CAD build for the part. Positions are in the model's coordinates, mm. A direction names the side the tool comes from. Give positions to 0.01 mm unless a question says otherwise; leave off trailing zeros. Order: outer loops, then holes, each group sorted by start corner. A loop starts at its lowest first (then second) coordinate and runs counter-clockwise, first axis right, second up. Notation, with made-up numbers: M 5,-27.75 L 21,-27.75 A20 cw 21,-12.75 Z; hole C 35.25,65 d6. An arc over 180 degrees is marked long. Put each result on its own line as item: value. Start each with the question number.
1) Pin check, flat tips, straight feed: pin 1 (1.6 mm diameter, centred on x = 5, z = 4.5, fed in from -Y); pin 2 (0.9 mm diameter, centred on x = -0.5, y = 3, fed in from +Z); pin 3 (3 mm diameter, centred on x = 6.5, z = 0.5, fed in from -Y). Stop position of each tip, or through.
2) Tool access for faces 5 (the face through (4.075, 2, 5)), 6 (the face through (3.6, 4.8, 4.8)), 7 (the face through (3.075, 2, 5)), 8 (the face through (6.55, 2, -1)): list every direction of +Z, -Z, +X, -X, +Y, -Y with a clear straight run to the whole face (end or side of a thin tool).
3) Two-plate mould, pull along Y, no slides. Class faces 1 (the face through (2, 2.3, 5)), 2 (the face through (7, 2, -2.95)), 3 (the face through (4, 4, 2)), 4 (the face through (3.358, 1.824, -1.574)): released by +Y, released by -Y, zero draft, split by the parting line, or undercut.
4) Cut at D-D (z = 4). Write the cut outline in (x, y) (3 decimals), and give its area (3 significant figures).
5) Cut at B-B (y = 2.8). Write the cut outline in (x, z) (3 decimals), and give its area (3 significant figures).
6) Drill centre lines: line 1 (X direction, y = 2.8, z = 1.45) (3 decimals); line 2 (X direction, y = 4.75, z = -0.5); line 3 (Z direction, x = 1, y = 4.75). Where is each one in solid material? Low to high. Write a range as [from, to].
7) Cut at C-C (x = 6.75). Write the cut outline in (y, z).
8) Cut at A-A (z = 0.25). Write the cut outline in (x, y) (3 decimals).
Autodesk Fusion 360 part; units mm, degrees
sketch "Sketch1" plane through (0, 0, 0) normal (0, 1, 0) x (1, 0, 0)
  line L0 (0, 0) -> (7.15, 0)
  line L1 (7.15, 0) -> (7.15, -3.3)
  line L2 (7.15, -3.3) -> (0, -3.3)
  line L3 (0, -3.3) -> (0, 0)
  line L4 (0, 0) -> (0.6, 0)
  line L5 (0.6, 0) -> (0.6, 2.95)
  line L6 (0.6, 2.95) -> (0, 2.95)
  line L7 (0, 2.95) -> (0, 0)
  line L8 (7.15, 0) -> (6.55, 0)
  line L9 (6.55, 0) -> (6.55, 2.95)
  line L10 (6.55, 2.95) -> (7.15, 2.95)
  line L11 (7.15, 2.95) -> (7.15, 0)
  dimension "d1" = 7.15
  dimension "d2" = 3.3
  dimension "d3" = 0.6
  dimension "d4" = 2.95
  dimension "d5" = 0.6
  dimension "d6" = 2.95
extrude "Extrude1" add sketch "Sketch1" along normal blind 5.6
sketch "Sketch2" plane through (7.15, 0, 0) normal (1, 0, 0) x (0, 1, 0)
  line L0 (0, 3.3) -> (0, -2.95)
  line L1 (0, -2.95) -> (5.6, -2.95)
  line L2 (5.6, -2.95) -> (5.6, 3.3)
  line L3 (5.6, 3.3) -> (0, 3.3)
  line L4 (1.675, -2.95) -> (3.925, -2.95)
  line L5 (3.925, -2.95) -> (3.925, 2.05)
  line L6 (3.925, 2.05) -> (1.675, 2.05)
  line L7 (1.675, 2.05) -> (1.675, -2.95)
  point P0 (2.8, 0)
  dimension "d12" = 2.25
  dimension "d13" = 5
extrude "Extrude2" add sketch "Sketch2" along normal blind 0.8 contours L1 L4 L5 L6 L7
sketch "Sketch3" plane through (0, 0, 0) normal (-1, 0, 0) x (0, -1, 0)
  line L0 (0, -2.95) -> (0, 3.3)
  line L1 (0, 3.3) -> (-5.6, 3.3)
  line L2 (-5.6, 3.3) -> (-5.6, -2.95)
  line L3 (-5.6, -2.95) -> (0, -2.95)
  line L4 (-1.675, -2.5004) -> (-1.675, -2.95)
  line L5 (-1.675, -2.95) -> (-3.925, -2.95)
  line L6 (-3.925, -2.95) -> (-3.925, -2.5004)
  line L7 (-1.675, -2.95) -> (-3.925, -2.95)
  line L8 (-3.925, -2.95) -> (-3.925, 2.05)
  line L9 (-3.925, 2.05) -> (-1.675, 2.05)
  line L10 (-1.675, 2.05) -> (-1.675, -2.95)
  point P0 (-2.8, -0.0004)
  dimension "d19" = 2.25
  dimension "d20" = 5
extrude "Extrude3" add sketch "Sketch3" along normal blind 0.8 contours L3 L4 L5 L6 L7 L8 L9 L10
sketch "Sketch4" plane through (0, 0, 0) normal (0, -1, 0) x (1, 0, 0)
  line L0 (0.6, -2.95) -> (0.6, 0)
  line L1 (0.6, 0) -> (6.55, 0)
  line L2 (6.55, 0) -> (6.55, -2.95)
  line L3 (6.55, -2.95) -> (7.15, -2.95)
  line L4 (7.15, -2.95) -> (7.15, 3.3)
  line L5 (7.15, 3.3) -> (0, 3.3)
  line L6 (0, 3.3) -> (0, -2.95)
  line L7 (0, -2.95) -> (0.6, -2.95)
  line L8 (0, 0) -> (0.6, 0)
  line L9 (0.6, 0) -> (0.6, -2.95)
  line L10 (0.6, -2.95) -> (0, -2.95)
  line L11 (0, -2.95) -> (0, 0)
  line L12 (6.55, 0) -> (7.15, 0)
  line L13 (7.15, 0) -> (7.15, -2.95)
  line L14 (7.15, -2.95) -> (6.55, -2.95)
  line L15 (6.55, -2.95) -> (6.55, 0)
extrude "Extrude4" add sketch "Sketch4" along normal blind 2 contours L0 L6 L7 L8 L9 L10 L11 | L2 L3 L4 L12 L13 L14 L15
sketch "Sketch5" plane through (0, 0, 0) normal (-1, 0, 0) x (0, -1, 0)
  line L0 (-3.925, -2.95) -> (-3.925, 2.05)
  line L1 (-3.925, 2.05) -> (-1.675, 2.05)
  line L2 (-1.675, 2.05) -> (-1.675, -2.95)
  line L3 (0, 0) -> (0, 3.3)
  line L4 (0, 3.3) -> (-5.6, 3.3)
  line L5 (-5.6, 3.3) -> (-5.6, -2.95)
  line L6 (-5.6, -2.95) -> (-3.925, -2.95)
sketch "Sketch6" plane through (0, 0, -2.95) normal (0, 0, -1) x (1, 0, 0)
  line L0 (0, 2) -> (0, -1.675)
  line L1 (0, -1.675) -> (-0.8, -1.675)
  line L2 (-0.8, -1.675) -> (-0.8, -3.925)
  line L3 (-0.8, -3.925) -> (0, -3.925)
  line L4 (0, -3.925) -> (0, -5.6)
  line L5 (0, -5.6) -> (0.6, -5.6)
  line L6 (0.6, -5.6) -> (0.6, 2)
  line L7 (0.6, 2) -> (0, 2)
  line L8 (0.6, 2) -> (0, 2)
  line L9 (0, 2) -> (0, 1.4)
  line L10 (0, 1.4) -> (0.6, 1.4)
  line L11 (0.6, 1.4) -> (0.6, 2)
sketch "Sketch7" plane through (0, 0, -2.95) normal (0, 0, -1) x (1, 0, 0)
  line L0 (6.55, 2) -> (6.55, -5.6)
  line L1 (6.55, -5.6) -> (7.15, -5.6)
  line L2 (7.15, -5.6) -> (7.15, -3.925)
  line L3 (7.15, -3.925) -> (7.95, -3.925)
  line L4 (7.95, -3.925) -> (7.95, -1.675)
  line L5 (7.95, -1.675) -> (7.15, -1.675)
  line L6 (7.15, -1.675) -> (7.15, 2)
  line L7 (7.15, 2) -> (6.55, 2)
  line L8 (7.15, 2) -> (6.55, 2)
  line L9 (6.55, 2) -> (6.55, 1.4)
  line L10 (6.55, 1.4) -> (7.15, 1.4)
  line L11 (7.15, 1.4) -> (7.15, 2)
  dimension "d25" = 0.6
extrude "Extrude5" add sketch "Sketch7" sketch "Sketch6" along normal blind 0.5 contours L0 L6 L7 L8 L9 L10 L11 of sketch 2 contours L0 L6 L7 L8 L9 L10 L11
sketch "Sketch8" plane through (0, 0, 0) normal (-1, 0, 0) x (0, -1, 0)
  line L0 (0.2, 0) -> (1.25, -2.95)
  line L1 (1.25, -2.95) -> (1.3, -3.6)
  line L2 (1.3, -3.6) -> (2.5, -3.6)
  line L3 (2.5, -3.6) -> (2.5, 0.457)
  line L4 (2.5, 0.457) -> (0.2, 0)
sketch "Sketch9" plane through (0, -1.35, -1.5715) normal (-1, 0, 0) x (0, -1, 0)
extrude "Extrude6" cut sketch "Sketch8" against normal blind 11
sketch "Sketch10" plane through (0, 0, 0) normal (0, 0, -1) x (1, 0, 0)
  line L0 (6.55, 0) -> (0.6, 0)
  line L1 (0.6, 0) -> (0.6, -5.6)
  line L2 (0.6, -5.6) -> (6.55, -5.6)
  line L3 (6.55, -5.6) -> (6.55, 0)
  line L4 (3.575, -5.6) -> (3.575, 0)
  circle A0 centre (3.575, -2.8) radius 1
  circle A1 centre (3.575, -2.8) radius 2
  dimension "d30" = 2
  dimension "d31" = 4
extrude "Extrude7" cut sketch "Sketch10" against normal blind 2 contours L4 A0 A1 | L4 A0 A1
extrude "Extrude8" add 1 faces at (3.8935, 2.8983, 0) along direction (0, 0, -1) blind 5.5
sketch "Sketch11" plane through (0, 0, 0) normal (0, 1, 0) x (1, 0, 0)
fillet "Fillet1" radius 0.25 1 edges at (2.6427, 3.1616, -5.5)
sketch "Sketch12" plane through (0, 0, 3.3) normal (0, 0, 1) x (-1, 0, 0)
  line L0 (0, 0) -> (-7.15, 0)
  line L1 (-7.15, 0) -> (-7.15, -5.6)
  line L2 (-7.15, -5.6) -> (0, -5.6)
  line L3 (0, -5.6) -> (0, 0)
  line L4 (-3.575, -5.6) -> (-3.575, 0)
  line L5 (0, -2.8) -> (-7.15, -2.8)
  line L6 (-1.575, -4.8) -> (-5.575, -4.8)
  line L7 (-5.575, -4.8) -> (-5.575, -0.8)
  line L8 (-5.575, -0.8) -> (-1.575, -0.8)
  line L9 (-1.575, -0.8) -> (-1.575, -4.8)
  line L10 (-1.575, -4.8) -> (-5.575, -0.8) construction
  line L11 (-5.575, -4.8) -> (-1.575, -0.8) construction
  line L12 (-3.075, -4.8) -> (-4.075, -4.8)
  line L13 (-4.075, -4.8) -> (-4.075, -0.8)
  line L14 (-4.075, -0.8) -> (-3.075, -0.8)
  line L15 (-3.075, -0.8) -> (-3.075, -4.8)
  line L16 (-3.075, -4.8) -> (-4.075, -0.8) construction
  line L17 (-4.075, -4.8) -> (-3.075, -0.8) construction
  line L18 (-1.575, -3.3) -> (-5.575, -3.3)
  line L19 (-5.575, -3.3) -> (-5.575, -2.3)
  line L20 (-5.575, -2.3) -> (-1.575, -2.3)
  line L21 (-1.575, -2.3) -> (-1.575, -3.3)
  line L22 (-1.575, -3.3) -> (-5.575, -2.3) construction
  line L23 (-5.575, -3.3) -> (-1.575, -2.3) construction
  point P0 (-3.575, -2.8)
  point P1 (-3.575, -2.8)
  point P2 (-3.575, -2.8)
  dimension "d38" = 4
  dimension "d39" = 4
  dimension "d40" = 1
  dimension "d41" = 4
  dimension "d42" = 4
  dimension "d43" = 1
extrude "Extrude9" add sketch "Sketch12" along normal blind 3 contours L4 L8 L14 L15 L20 | L4 L8 L13 L14 L20 | L5 L9 L15 L18 L21 | L5 L9 L15 L20 L21 | L4 L5 L15 L20 | L4 L5 L13 L20 | L4 L5 L15 L18 | L5 L7 L13 L19 L20 | L5 L7 L13 L18 L19 | L4 L5 L13 L18 | L4 L6 L12 L13 L18 | L4 L6 L12 L15 L18
sketch "Sketch13" plane through (0, 0, 0) normal (1, 0, 0) x (0, 1, 0)
sketch "Sketch14" plane through (0, 0, -5.5) normal (0, 0, -1) x (1, 0, 0)
  circle A0 centre (3.575, -2.8) radius 0.75
sketch "Sketch15" plane through (7.95, 0, 0) normal (1, 0, 0) x (0, 1, 0)
  line L0 (1.675, 2.05) -> (1.675, -2.95)
  line L1 (1.675, -2.95) -> (3.925, -2.95)
  line L2 (3.925, -2.95) -> (3.925, 2.05)
  line L3 (3.925, 2.05) -> (1.675, 2.05)
  line L4 (0.8, 6.3) -> (4.8, 6.3)
  line L5 (0.8, 6.3) -> (0.8, 3.3)
  line L6 (0, 3.3) -> (5.6, 3.3)
  line L7 (5.6, 3.3) -> (5.6, -2.95)
  line L8 (5.6, -2.95) -> (5.6, 3.3)
  line L9 (-1.25, -2.95) -> (5.6, -2.95)
  line L10 (0, 0) -> (0, -2.95)
  dimension "d46" = 4
  dimension "d47" = 3
  dimension "d48" = 5.6
  dimension "d49" = 6.25
  dimension "d50" = 6.85
  dimension "d51" = 2.95
Solution:
1. pin 1: y = 2.3
1. pin 2: z = 2.05
1. pin 3: y = -0.56
2. face 5: +Z, +X, -Y
2. face 6: +Z, +X, -X, +Y
2. face 7: +Z, -X, -Y
2. face 8: -Z, +Y, -Y
3. face 1: released by -Y
3. face 2: zero draft
3. face 3: undercut
3. face 4: undercut
4. outline: M 1.575,2.3 L 3.075,2.3 L 3.075,0.8 L 4.075,0.8 L 4.075,2.3 L 5.575,2.3 L 5.575,3.3 L 4.075,3.3 L 4.075,4.8 L 3.075,4.8 L 3.075,3.3 L 1.575,3.3 Z
4. area: 7.00 mm²
5. outline: M -0.8,-2.95 L 0.6,-2.95 L 0.6,0 L 1.575,0 L 1.575,2 L 2.575,2 L 2.575,-5.25 A0.25 ccw 2.825,-5.5 L 4.325,-5.5 A0.25 ccw 4.575,-5.25 L 4.575,2 L 5.575,2 L 5.575,0 L 6.55,0 L 6.55,-2.95 L 7.95,-2.95 L 7.95,2.05 L 7.15,2.05 L 7.15,3.3 L 5.575,3.3 L 5.575,6.3 L 1.575,6.3 L 1.575,3.3 L 0,3.3 L 0,2.05 L -0.8,2.05 Z
5. area: 54.1 mm²
6. line 1: [-0.8, 1.575], [2.575, 4.575], [5.575, 7.95]
6. line 2: [0, 0.6], [6.55, 7.15]
6. line 3: [0, 3.3]
7. outline: M -1.25,-2.95 L 5.6,-2.95 L 5.6,3.3 L 0,3.3 L 0,0 L -0.2,0 Z
8. outline: M -0.8,1.675 L 0,1.675 L 0,0 L 7.15,0 L 7.15,1.675 L 7.95,1.675 L 7.95,3.925 L 7.15,3.925 L 7.15,5.6 L 0,5.6 L 0,3.925 L -0.8,3.925 Z; C 3.575,2.8 d2; hole C 3.575,2.8 d4
